Input: part model. Units: mm. Frame: model coordinates. Face numbers are marked on the shaded views. A direction names the side the tool comes from. Round coordinates to 2 decimals unless told otherwise and drop trailing zeros. Write each loop counter-clockwise with the first axis right and the second up, starting at its lowest first coordinate (ties: lowest second). Pieces come first, ordered by that corner, then holes. Notation, with made-up numbers: (-31, 74.25) -> (-16, 74.25) arc R11 cw to (-16, 90.25) -> close; hole circle Ø11 at (64, 8.5). An arc over 180 degrees is marked (long way). Use CSV: the item, a comma, the result in double quotes.
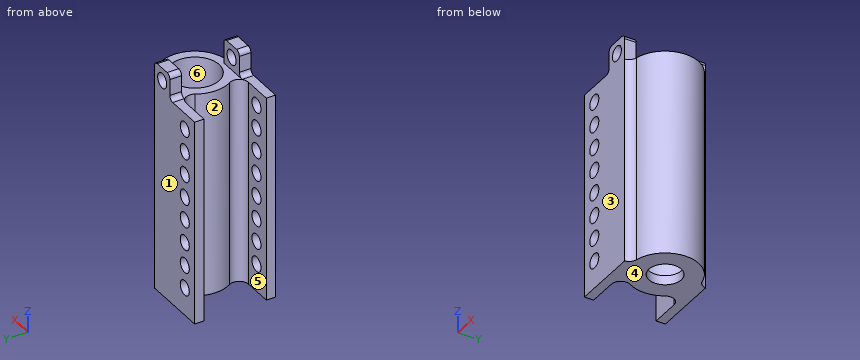
Autodesk Inventor part; units mm, degrees
ref_plane "YZ Plane" through (0, 0, 0) normal (1, 0, 0) x (0, 1, 0)
ref_plane "XZ Plane" through (0, 0, 0) normal (0, 1, 0) x (-1, 0, 0)
ref_plane "XY Plane" through (0, 0, 0) normal (0, 0, 1) x (1, 0, 0)
sketch "Sketch1" plane through (0, 0, 0) normal (0, 0, 1) x (1, 0, 0)
  circle A0 centre (0, 0) radius 5.25
  circle A1 centre (0, 0) radius 7.25
  dimension "d0" = 10.5
  dimension "d1" = 2
extrude "Extrusion1" add sketch "Sketch1" along normal blind 42.5
extrude "Extrusion2" add sketch "Sketch1" against normal blind 2 contours A0 | A1
sketch "Sketch2" plane through (0, 0, -2) normal (0, 0, -1) x (-1, 0, 0)
  circle A0 centre (0, 0) radius 7.25 construction
  circle A1 centre (0, 0) radius 3.5
  dimension "d6" = 7
extrude "Extrusion3" cut sketch "Sketch2" against normal through all
sketch "Sketch3" plane through (0, 0, 42.5) normal (0, 0, 1) x (1, 0, 0)
  circle A0 centre (0, 0) radius 7.25 construction
  circle A1 centre (0, 0) radius 5.25 construction
  line L0 (0, 0) -> (-18.4312, 0) construction
  circle A2 centre (0, 0) radius 7.25 construction
  line L1 (-2.6458, 6.75) -> (-14.25, 6.75) construction
  line L2 (-14.25, 6.75) -> (-14.25, -6.75) construction
  line L3 (-14.25, -6.75) -> (-2.6458, -6.75) construction
  line L4 (-2.6458, -6.75) -> (-2.6458, 6.75) construction
  line L5 (-7.25, 0) -> (-7.25, 11.3017) construction
  line L6 (-14.25, 6.75) -> (0, 6.75)
  line L7 (0, 6.75) -> (0, 8.75)
  line L8 (0, 8.75) -> (-14.25, 8.75)
  line L9 (-14.25, 8.75) -> (-14.25, 6.75)
  dimension "d9" = 7
  dimension "d10" = 13.5
  dimension "d11" = 2
  dimension "d16" = 0
extrude "Extrusion4" add sketch "Sketch3" against normal up to surface (44.5 mm away)
ref_plane "Work Plane1" through (0, 0, 42.5) normal (0, 1, 0) x (1, 0, 0)
mirror "Mirror1" about plane through (0, 0, 42.5) normal (0, 1, 0) of "Extrusion4"
fillet "Fillet1" radius 2 2 edges at (0, 7.25, 20.25) (0, -7.25, 20.25)
fillet "Fillet2" radius 2 2 edges at (-2.6458, 6.75, 20.25) (-2.6458, -6.75, 20.25)
sketch "Sketch4" plane through (-14.25, -8.75, -2) normal (0, -1, 0) x (1, 0, 0)
  line L0 (0, 0) -> (14.25, 0) construction
  line L1 (14.25, 44.5) -> (14.25, 0) construction
  line L2 (14.25, 44.5) -> (0, 44.5) construction
  line L3 (0, 44.5) -> (0, 0) construction
  line L4 (3.5, 56.7252) -> (3.5, -16.7448) construction
  circle A0 centre (3.5, 6) radius 1.6
  line L5 (3.5, 61.7252) -> (3.5, -11.7448) construction
  circle A1 centre (3.5, 11) radius 1.6
  line L6 (3.5, 66.7252) -> (3.5, -6.7448) construction
  circle A2 centre (3.5, 16) radius 1.6
  line L7 (3.5, 71.7252) -> (3.5, -1.7448) construction
  circle A3 centre (3.5, 21) radius 1.6
  line L8 (3.5, 76.7252) -> (3.5, 3.2552) construction
  circle A4 centre (3.5, 26) radius 1.6
  line L9 (3.5, 81.7252) -> (3.5, 8.2552) construction
  circle A5 centre (3.5, 31) radius 1.6
  line L10 (3.5, 86.7252) -> (3.5, 13.2552) construction
  circle A6 centre (3.5, 36) radius 1.6
  line L11 (3.5, 91.7252) -> (3.5, 18.2552) construction
  circle A7 centre (3.5, 41) radius 1.6
  point P0 (14.25, 2)
  dimension "d19" = 3.5
  dimension "d20" = 3.2
  dimension "d21" = 6
  dimension "d24" = 5
extrude "Extrusion5" cut sketch "Sketch4" against normal through all
sketch "Sketch5" plane through (0, 0, 42.5) normal (0, 0, 1) x (1, 0, 0)
  arc A0 (1.5515, -7.082) -> (1.5515, 7.082) centre (0, 0) ccw construction
  arc A1 (0, 8.75) -> (1.5515, 7.082) centre (1.9795, 9.0357) ccw construction
  line L0 (0, 8.75) -> (-14.25, 8.75) construction
  line L1 (-14.25, 8.75) -> (-14.25, 6.75) construction
  line L2 (-14.25, 6.75) -> (-7.9373, 6.75) construction
  arc A2 (-6.2211, 3.723) -> (-7.9373, 6.75) centre (-7.9373, 4.75) ccw construction
  arc A3 (-6.2211, 3.723) -> (-6.2211, -3.723) centre (0, 0) ccw construction
  arc A4 (-7.9373, -6.75) -> (-6.2211, -3.723) centre (-7.9373, -4.75) ccw construction
  line L3 (-14.25, -6.75) -> (-7.9373, -6.75) construction
  line L4 (-14.25, -8.75) -> (-14.25, -6.75) construction
  line L5 (0, -8.75) -> (-14.25, -8.75) construction
  arc A5 (1.5515, -7.082) -> (0, -8.75) centre (1.9795, -9.0357) ccw construction
  circle A6 centre (0, 0) radius 5.25 construction
  line L6 (0, 8.75) -> (-14.25, 8.75)
  line L7 (0, 8.75) -> (-5.5, 8.75)
  line L8 (-5.5, 8.75) -> (-5.5, 6.25)
  line L9 (-5.5, 6.25) -> (0, 6.25)
  line L10 (0, 6.25) -> (0, 8.75)
  dimension "d31" = 2.5
  dimension "d32" = 5.5
extrude "Extrusion6" add sketch "Sketch5" along normal blind 5.5
mirror "Mirror2" about plane through (0, 0, 42.5) normal (0, 1, 0) of "Extrusion6"
sketch "Sketch6" plane through (-14.25, 8.75, 42.5) normal (0, 1, 0) x (1, 0, 0)
  circle A0 centre (3.5, 8.5) radius 1.6 construction
  circle A1 centre (3.5, 18.5) radius 1.6 construction
  circle A2 centre (3.5, 28.5) radius 1.6 construction
  circle A3 centre (3.5, 38.5) radius 1.6 construction
  circle A4 centre (3.5, 33.5) radius 1.6 construction
  circle A5 centre (3.5, 23.5) radius 1.6 construction
  circle A6 centre (3.5, 13.5) radius 1.6 construction
  circle A7 centre (3.5, 3.5) radius 1.6 construction
  line L0 (0, 44.5) -> (14.25, 44.5) construction
  line L1 (0, 0) -> (0, 44.5) construction
  line L2 (8.75, 0) -> (0, 0) construction
  line L3 (8.75, 0) -> (8.75, -5.5) construction
  line L4 (14.25, -5.5) -> (8.75, -5.5) construction
  line L5 (14.25, 0) -> (14.25, -5.5) construction
  line L6 (14.25, 0) -> (14.25, 44.5) construction
  line L7 (14.25, 0) -> (14.25, 44.5) construction
  line L8 (14.25, 0) -> (8.75, -5.5) construction
  line L9 (8.75, -5.5) -> (14.25, -5.5) construction
  line L10 (14.25, -5.5) -> (8.75, 0) construction
  circle A8 centre (11.5, -2.75) radius 1.6
  point P0 (14.25, 42.5)
  dimension "d35" = 3.2
extrude "Extrusion7" cut sketch "Sketch6" against normal through all
fillet "Fillet3" radius 1 6 edges at (-5.5, 7.5, 42.5) (-5.5, 7.5, 48) (0, 7.5, 48) (-5.5, -7.5, 42.5) (-5.5, -7.5, 48) (0, -7.5, 48)
properties part number "magnet-holder"
Item 1: Section query B-B on x = -2.75. Return the cut outline in (y, z).
Worked answers:
outline,"(-8.75, -2) -> (-2.17, -2) -> (-2.17, 0) -> (-4.47, 0) -> (-4.47, 42.5) -> (-6.25, 42.5) -> (-6.25, 43.65) -> (-8.75, 43.65) -> close; (-8.75, 46.85) -> (-6.25, 46.85) -> (-6.25, 48) -> (-8.75, 48) -> close; (2.17, -2) -> (8.75, -2) -> (8.75, 43.65) -> (6.25, 43.65) -> (6.25, 42.5) -> (4.47, 42.5) -> (4.47, 0) -> (2.17, 0) -> close; (6.25, 46.85) -> (8.75, 46.85) -> (8.75, 48) -> (6.25, 48) -> close"
Item 2: Section query D-D on x = -10.75. Give the number of separate pieces and of enclosed holes in the cut face, plus the area to 3 significant figures.
Worked answers:
separate pieces,"18"
enclosed holes,"0"
area,"75.6 mm²"
Item 3: Section query A-A on z = 34. Return the cut outline in (x, y).
Worked answers:
outline,"(-14.25, -8.75) -> (-12.35, -8.75) -> (-12.35, -6.75) -> (-14.25, -6.75) -> close; (-14.25, 6.75) -> (-12.35, 6.75) -> (-12.35, 8.75) -> (-14.25, 8.75) -> close; (-9.15, -8.75) -> (0, -8.75) arc R2 cw to (1.55, -7.08) arc R7.25 ccw to (1.55, 7.08) arc R2 cw to (0, 8.75) -> (-9.15, 8.75) -> (-9.15, 6.75) -> (-7.94, 6.75) arc R2 cw to (-6.22, 3.72) arc R7.25 ccw to (-6.22, -3.72) arc R2 cw to (-7.94, -6.75) -> (-9.15, -6.75) -> close; hole circle Ø10.5 at (0, 0)"
Item 4: First-contact query: pin 1 Ø3 at (x, z) = (5, 35.5) entering from +Y; pin 2 Ø3 at (y, z) = (8, 45.5) entering from +X; pin 3 Ø1 at (y, z) = (-4, 33.5) entering from -X. Flat tips, straight axial feed; report the tip coordinate or a pass-through.
Worked answers:
pin 1,"stops at y = 6.35"
pin 2,"stops at x = 0"
pin 3,"stops at x = -6.35"
Item 5: Line query: line 1 (Z direction, x = -2.75, y = -7.1); line 2 (Y direction, x = -11.25, z = 42); line 3 (Y direction, x = -6.5, z = 17). Output: solid intervals per line, ascending.
Worked answers:
line 1,"z = -2 to 43.65, 46.85 to 48"
line 2,"y = -8.75 to -6.75, 6.75 to 8.75"
line 3,"y = -8.75 to -6.14, -3.21 to 3.21, 6.14 to 8.75"
Item 6: Set-up query: the marked faces 4, 5 and 6. Return all of +Z, -Z, +X, -X, +Y, -Y with unobstructed straight access to the full face (end or side cutting, diameter ignored); none if empty.
Worked answers:
face 4,"-Z, +X, -X, +Y, -Y"
face 5,"+Z, -Z, -X"
face 6,"+Z"
Item 7: Section query C-C on z = 3.5. Return the cut outline in (x, y), plus the area to 3 significant figures.
Worked answers:
outline,"(-14.25, -8.75) -> (-12.27, -8.75) -> (-12.27, -6.75) -> (-14.25, -6.75) -> close; (-14.25, 6.75) -> (-12.27, 6.75) -> (-12.27, 8.75) -> (-14.25, 8.75) -> close; (-9.23, -8.75) -> (0, -8.75) arc R2 cw to (1.55, -7.08) arc R7.25 ccw to (1.55, 7.08) arc R2 cw to (0, 8.75) -> (-9.23, 8.75) -> (-9.23, 6.75) -> (-7.94, 6.75) arc R2 cw to (-6.22, 3.72) arc R7.25 ccw to (-6.22, -3.72) arc R2 cw to (-7.94, -6.75) -> (-9.23, -6.75) -> close; hole circle Ø10.5 at (0, 0)"
area,"131 mm²"
Item 8: Pull-direction query (Y, two-part tool) for the marked faces 1, 2 and 3; classes: +Y half, -Y half, draft (parallel to the pull), parting line (faces both ways), or undercut.
Worked answers:
face 1,"+Y half"
face 2,"undercut"
face 3,"-Y half"
